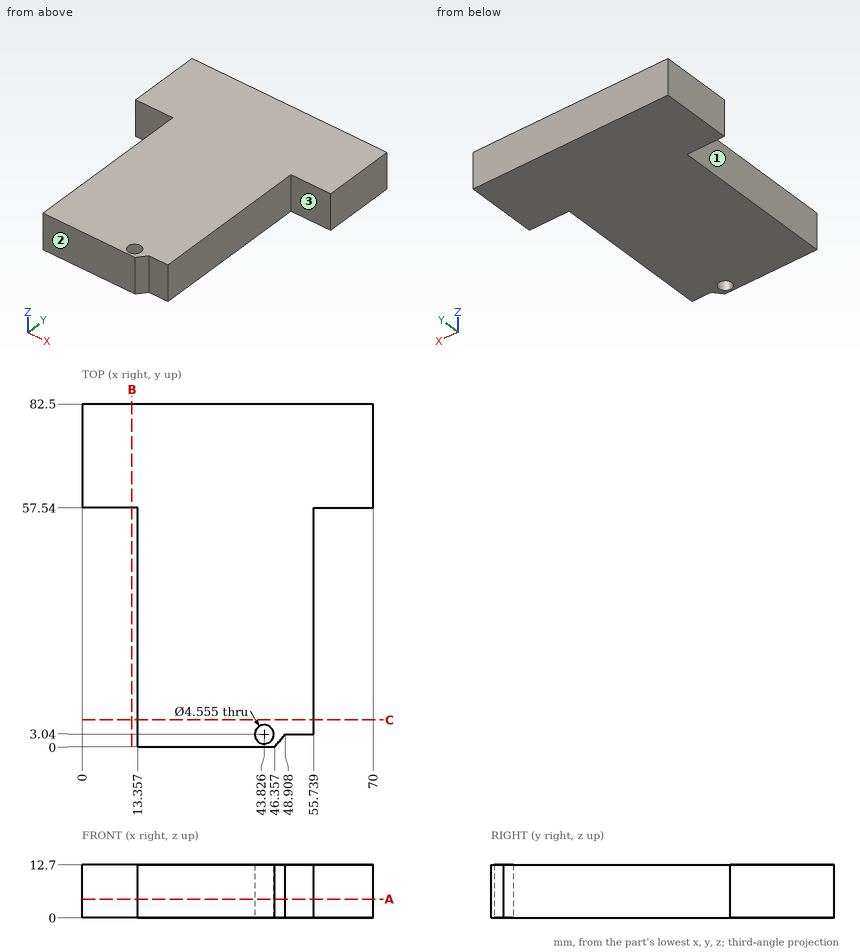
Verification items for this drawing (mm, ordinates from the low corner). A direction names the side the tool comes from. Round coordinates to 2 decimals unless told otherwise and drop trailing zeros. Write each loop counter-clockwise with the first axis right and the second up, starting at its lowest first coordinate (ties: lowest second). Pieces come first, ordered by that corner, then holes. Notation, with made-up numbers: M 63.25,29.5 L 119.25,29.5 A10 ccw 119.25,33.5 Z; hole C 4.5,-19.5 d3. An arc over 180 degrees is marked long. Write item = value, one per line. Start each with the question number.
1. Section check C-C, the plane y = 6.5. Record the cut outline in (x, z), then the cut area to 3 significant figures.
2. Scan lines: line 1 (X direction, y = 13, z = 6); line 2 (Y direction, x = 5, z = 9); line 3 (Y direction, x = 53, z = 3.25). Record each from-to range of solid material in increasing order. Write a range as [from, to].
3. Gauge pin test, flat ends, axial feed: pin 1 (5 mm diameter, centred on y = 32, z = 6.5, fed in from +X); pin 2 (4 mm diameter, centred on x = 43.83, y = 3.04, fed in from +Z); pin 3 (5.5 mm diameter, centred on x = 53, z = 7.5, fed in from -Y); pin 4 (4 mm diameter, centred on x = 6, z = 5.5, fed in from -Y). Record the tip position at first contact, or that the pin passes through.
4. Section check B-B, the plane x = 12. Record the cut outline in (y, z).
5. Tool access check on the marked faces 1, 2 and 3. Record the directions out of +Z, -Z, +X, -X, +Y, -Y that give a thin tool (end or side, any length) a straight path to the whole face; none if there is none.
6. Section check A-A, the plane z = 4.5. Record the cut outline in (x, y) (1 decimal), then the cut area to 4 significant figures.
Results found:
q1.outline = M 13.36,0 L 55.74,0 L 55.74,12.7 L 13.36,12.7 Z
q1.area = 538 mm^2
q2.line_1 = [13.36, 55.74]
q2.line_2 = [57.54, 82.5]
q2.line_3 = [3.04, 82.5]
q3.pin_1 = 55.74
q3.pin_2 = through
q3.pin_3 = 3.04
q3.pin_4 = 57.54
q4.outline = M 57.54,0 L 82.5,0 L 82.5,12.7 L 57.54,12.7 Z
q5.face_1 = +Z, -Z, -X, -Y
q5.face_2 = +Z, -Z, +X, -X, -Y
q5.face_3 = +Z, -Z, +X, -Y
q6.outline = M 0,57.5 L 13.4,57.5 L 13.4,0 L 46.4,0 L 48.9,3 L 55.7,3 L 55.7,57.5 L 70,57.5 L 70,82.5 L 0,82.5 Z; hole C 43.8,3 d4.6
q6.area = 4,145 mm^2
